Source: CAD feature listing. Evaluate the final solid. Frame: model axes, mm. A direction names the side the tool comes from. Give positions to 0.01 mm unless a question says otherwise; leave off trailing zeros. Order: outer loops, then holes, each group sorted by start corner. A loop starts at its lowest first (then second) coordinate and runs counter-clockwise, first axis right, second up.
```python
from build123d import *

# Parameters (mm, degrees)
SKETCH1_R           = 9.25
BOSS_EXTRUDE1_DEPTH = 12
SKETCH2_R           = 3
CUT_EXTRUDE1_DEPTH  = 5.8
SKETCH3_R           = 14
CUT_EXTRUDE2_DEPTH  = 10
CUT_EXTRUDE3_DEPTH  = 74


with BuildPart() as part:
    # Sketch1 → Boss-Extrude1 (new body)
    with BuildSketch(Plane.XY):
        with BuildLine():
            Line((-36.5, 0), (36.5, 0))
            Line((36.5, 0), (36.5, 4.8))
            Line((36.5, 4.8), (23, 4.8))
            ThreePointArc((23, 4.8), (15.928932188, 7.728932188), (13, 14.8))
            Line((13, 14.8), (13, 35))
            ThreePointArc((13, 35), (0, 48), (-13, 35))
            Line((-13, 35), (-13, 14.8))
            ThreePointArc((-13, 14.8), (-15.928932188, 7.728932188), (-23, 4.8))
            Line((-23, 4.8), (-36.5, 4.8))
            Line((-36.5, 4.8), (-36.5, 0))
        make_face()
        with Locations((0, 35)):
            Circle(SKETCH1_R, mode=Mode.SUBTRACT)
    extrude(amount=BOSS_EXTRUDE1_DEPTH)

    # Sketch2 → Cut-Extrude1 (cut, through all)
    with BuildSketch(Plane(origin=(0, 4.8, 0), x_dir=(1, 0, 0), z_dir=(0, 1, 0))):
        with Locations(Location((-30, -6, 0), (0, 0, 180))):  # turned: the seam where the file's is
            Circle(SKETCH2_R)
        with Locations(Location((30, -6, 0), (0, 0, 180))):  # turned: the seam where the file's is
            Circle(SKETCH2_R)
    extrude(amount=-CUT_EXTRUDE1_DEPTH, mode=Mode.SUBTRACT)

    # Sketch3 → Cut-Extrude2 (cut)
    with BuildSketch(Plane.XY.offset(12)):
        with Locations((0, 35)):
            Circle(SKETCH3_R)
    extrude(amount=-CUT_EXTRUDE2_DEPTH, mode=Mode.SUBTRACT)

    # Sketch4 → Cut-Extrude3 (cut, through all)
    with BuildSketch(Plane.ZY.offset(36.5)):
        Polygon((2, 29.803847577), (12, 4.8), (12, 29.803847577), align=None)
    extrude(amount=-CUT_EXTRUDE3_DEPTH, mode=Mode.SUBTRACT)


solid = part.part
```
1) Section query A-A, the plane x = 0. Return the cut outline in (y, z).
Report:
outline: (0, 0) - (25.75, 0) - (25.75, 2) - (21, 2) - (21, 5.52) - (4.8, 12) - (0, 12) - close; (44.25, 0) - (48, 0) - (48, 2) - (44.25, 2) - close
2) Section query C-C, the plane y = 27. Return the cut outline in (x, z).
Report:
outline: (-13, 0) - (-4.64, 0) - (-4.64, 2) - (-11.49, 2) - (-11.49, 3.12) - (-13, 3.12) - close; (4.64, 0) - (13, 0) - (13, 3.12) - (11.49, 3.12) - (11.49, 2) - (4.64, 2) - close
3) Section query D-D, the plane y = 3. Return the cut outline in (x, z), and give its area (3 significant figures).
Report:
outline: (-36.5, 0) - (36.5, 0) - (36.5, 12) - (-36.5, 12) - close; hole circle Ø6 at (-30, 6); hole circle Ø6 at (30, 6)
area: 819 mm2
4) Draft query along X for faces 6 (the cylindrical face through (0, 21, 4)), 7 (the flat face through (-13, 23, 2)), 8 (the cylindrical face through (16.01, 7.65, 5.92)). Return one class per face: +X half, -X half, draft (parallel to the pull), parting line (faces both ways), or undercut.
Report:
face 6: undercut
face 7: -X half
face 8: +X half
5) Section query B-B, the plane z = 7.25. Return the cut outline in (x, y).
Report:
outline: (-36.5, 0) - (-32.73, 0) - (-32.73, 4.8) - (-36.5, 4.8) - close; (-27.27, 0) - (27.27, 0) - (27.27, 4.8) - (23, 4.8) arc R10 cw to (13, 14.8) - (13, 16.68) - (-13, 16.68) - (-13, 14.8) arc R10 cw to (-23, 4.8) - (-27.27, 4.8) - close; (32.73, 0) - (36.5, 0) - (36.5, 4.8) - (32.73, 4.8) - close
6) Pin query (flat end, axial travel): pin 1 (4 mm diameter, centred on x = -11.5, y = 6.5, fed in from -Z). Return the tip coordinate at first contact, or that it passes through.
Report:
pin 1: stops at z = 0
7) Material intervals for L1, parallel to X at y = 4.5, z = 8; L2, parallel to Z at x = -30, y = 2.25; L3, parallel to Y at x = 0, z = 1.45, sorted ascending.
Report:
L1: x = -36.5 to -32.24, -27.76 to 27.76, 32.24 to 36.5
L2: z = 0 to 3, 9 to 12
L3: y = 0 to 25.75, 44.25 to 48
8) Reachability of faces 1 (the cylindrical face through (-27, 2, 6)), 2 (the flat face through (-1, 2, 12)), 3 (the flat face through (3, 26, 2)), 4 (the flat face through (-26.7, 4.8, 5.9)), 5 (the flat face through (13, 23, 3)) from +Z, -Z, +X, -X, +Y, -Y: full face, straight path, thin tool, end or side. Return the list, or none.
Report:
face 1: +Y, -Y
face 2: +Z, +X, -X, +Y, -Y
face 3: +Z, +Y
face 4: +Z, -Z, -X, +Y
face 5: +Z, -Z, +X, +Y
